CAD build for the part. Positions are in the model's coordinates, mm. A direction names the side the tool comes from. Coordinates: 2 decimals unless noted, no trailing zeros. Order: outer loops, then holes, each group sorted by start corner. A loop starts at its lowest first (then second) coordinate and runs counter-clockwise, first axis right, second up. Notation, with made-up numbers: (-36.75, -9) - (9.25, -9) arc R18 cw to (9.25, 17) - close; hole circle Ø7 at (63.5, -28.5). An arc over 180 degrees is marked (long way). Use one line per item in the form item = value.
```python
from build123d import *

# Parameters (mm, degrees)
SKETCH1_R           = 12
BOSS_EXTRUDE1_DEPTH = 45
SKETCH2_R           = 7.5
BOSS_EXTRUDE2_DEPTH = 16
SKETCH3_W           = 53
SKETCH3_H           = 46
BOSS_EXTRUDE3_DEPTH = 17
CUT_EXTRUDE1_DEPTH  = 2


with BuildPart() as part:
    # Sketch1 → Boss-Extrude1 (new, symmetric)
    with BuildSketch(Plane.XY):
        with Locations(Location((0, 0, 0), (0, 0, 180))):
            Circle(SKETCH1_R)
    extrude(amount=BOSS_EXTRUDE1_DEPTH, both=True)

    # Sketch2 → Boss-Extrude2 (add)
    with BuildSketch(Plane(origin=(0, 0, 0), x_dir=(1, 0, 0), z_dir=(0, 1, 0))):
        with Locations(Location((0, 0, 0), (0, 0, 270))):
            Circle(SKETCH2_R)
    extrude(amount=-BOSS_EXTRUDE2_DEPTH)

    # Sketch3 → Boss-Extrude3 (add)
    with BuildSketch(Plane.XZ.offset(16)):
        with Locations((-14.5, 0)):
            Rectangle(SKETCH3_W, SKETCH3_H)
    extrude(amount=BOSS_EXTRUDE3_DEPTH)

    # Sketch4 → Cut-Extrude1 (cut)
    with BuildSketch(Plane(origin=(12, 0, 0), x_dir=(0, 0, -1), z_dir=(1, 0, 0))):
        with BuildLine():
            Line((-19.5, 6.5), (19.5, 6.5))
            ThreePointArc((19.5, 6.5), (26, 0), (19.5, -6.5))
            Line((19.5, -6.5), (-19.5, -6.5))
            ThreePointArc((-19.5, -6.5), (-26, 0), (-19.5, 6.5))
        make_face()
    extrude(amount=-CUT_EXTRUDE1_DEPTH, mode=Mode.SUBTRACT)


solid = part.part
```
Item 1: Drill centre lines: line 1 (Z direction, x = -18, y = -22); line 2 (Y direction, x = -13.5, z = -17.5); line 3 (Y direction, x = -6, z = -21.5). Where is each one in solid material? Low to high. Write a range as [from, to].
Derived:
line_1 = [-23, 23]
line_2 = [-33, -16]
line_3 = [-33, -16], [-10.39, 10.39]
Item 2: Cut at A-A, the plane z = 17.5. Write the cut outline in (x, y), plus the area to 3 significant figures.
Derived:
outline = (-41, -33) - (12, -33) - (12, -16) - (-41, -16) - close; (10, -6.5) - (10, 6.5) - (10.09, 6.5) arc R12 ccw (long way) to (10.09, -6.5) - close
area = 1,340 mm²
Item 3: Cut at B-B, the plane y = 0. Write the cut outline in (x, z), plus the area to 3 significant figures.
Derived:
outline = (-12, -45) - (12, -45) - (12, -26) - (10, -26) - (10, 26) - (12, 26) - (12, 45) - (-12, 45) - close
area = 2,060 mm²
Item 4: Cut at C-C, the plane z = 0. Write the cut outline in (x, y).
Derived:
outline = (-41, -33) - (12, -33) - (12, -16) - (7.5, -16) - (7.5, -9.37) arc R12 ccw to (10.09, -6.5) - (10, -6.5) - (10, 6.5) - (10.09, 6.5) arc R12 ccw (long way) to (-7.5, -9.37) - (-7.5, -16) - (-41, -16) - close
Item 5: 3-axis set-ups, long thin cutter, end or side, ignore diameter. For faces 4 (the face through (-41, -24, 0)), 5 (the face through (-2.87, -13.37, 6.93)), 6 (the face through (-15, -24, -23)), 7 (the face through (11, 0, 26)), 8 (the face through (-15, -24, 23)): which of +Z, -Z, +X, -X, +Y, -Y reach the whole face in a straight line?
Derived:
face_4 = +Z, -Z, -X, +Y, -Y
face_5 = none
face_6 = -Z, +X, -X, -Y
face_7 = +X
face_8 = +Z, +X, -X, -Y
Item 6: Two-plate mould, pull along X, no slides. Class faces 1 (the face through (10, 0, 0)), 2 (the face through (-11.085, 4.596, 0.63)), 3 (the face through (0, 0, 45)): +X half, -X half, draft (parallel to the pull), parting line (faces both ways), or undercut.
Derived:
face_1 = +X half
face_2 = parting line
face_3 = draft
Item 7: Cut at D-D, the plane x = 0. Write the cut outline in (y, z), plus the area to 3 significant figures.
Derived:
outline = (-33, -23) - (-16, -23) - (-16, -7.5) - (-12, -7.5) - (-12, -45) - (12, -45) - (12, 45) - (-12, 45) - (-12, 7.5) - (-16, 7.5) - (-16, 23) - (-33, 23) - close
area = 3,000 mm²
Item 8: Drop flat-ended pins along their axis: pin 1 (6 mm diameter, centred on x = 0.5, z = 29.5, fed in from -Y); pin 2 (3 mm diameter, centred on x = -15, z = -13.5, fed in from +Y); pin 3 (10 mm diameter, centred on x = -19.5, y = -25, fed in from +Z); pin 4 (4 mm diameter, centred on x = -1, z = -12, fed in from +Y). Give the stop position or say it passes through.
Derived:
pin_1 = -12
pin_2 = -16
pin_3 = 23
pin_4 = 12
